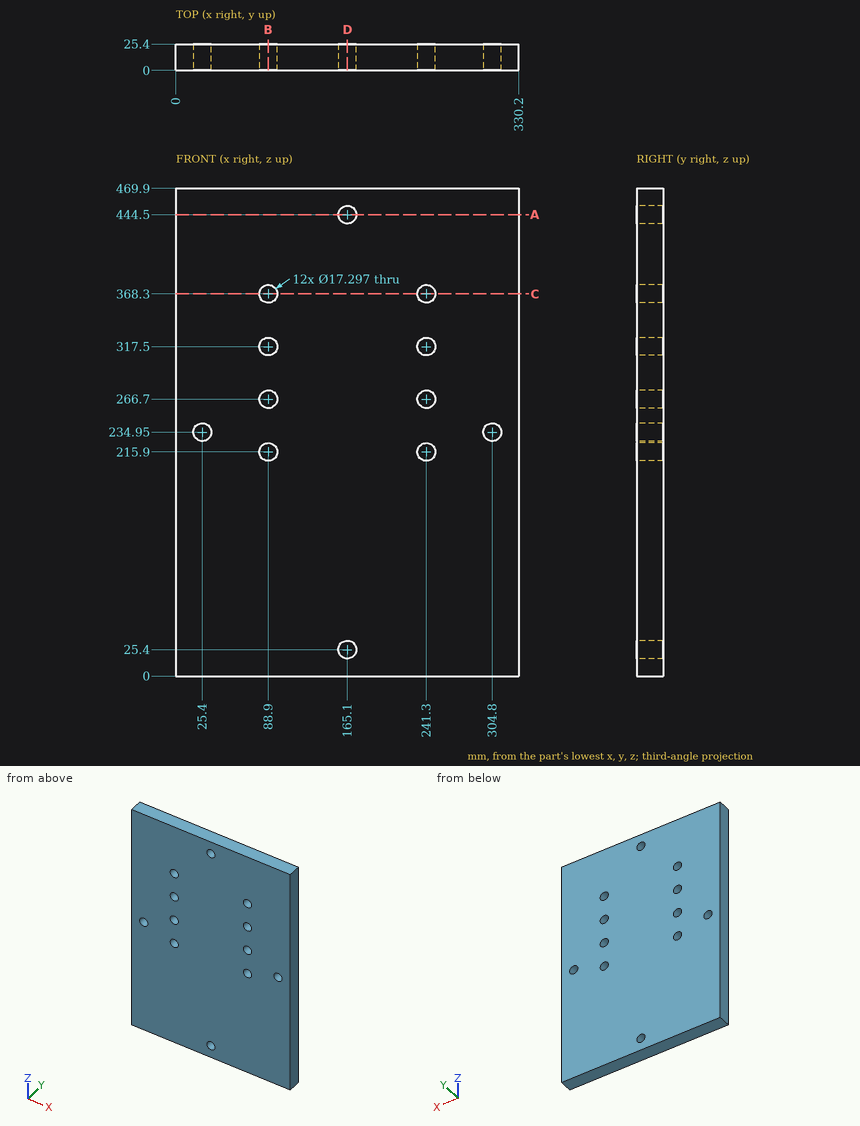
Geometry check sheet. Reference: drawing and pictorial views, mm from the part's lowest x, y, z. Round coordinates to 2 decimals unless told otherwise and drop trailing zeros. Order: outer loops, then holes, each group sorted by start corner. A loop starts at its lowest first (then second) coordinate and runs counter-clockwise, first axis right, second up. Notation, with made-up numbers: M 18.5,10.5 L 28.5,10.5 A27 cw 28.5,35.5 Z; hole C 74,-38 d4. An arc over 180 degrees is marked long. Answer in a Markdown table with one row per item.
(1) Go/stop test with flat-tipped pins: P1, Ø10.5, axis at x = 241.3, z = 215.9, coming from the +Y side; P2, Ø3, axis at x = 274.5, y = 20.5, coming from the -Z side. Record where each tip stops, or that it passes through.
Responses:
| item | result |
|---|---|
| P1 | passes through |
| P2 | stops at z = 0 |
(2) Sectioned sample at C-C, the plane z = 368.3. Record the cut outline in (x, y), and give its area (3 significant figures).
Responses:
| item | result |
|---|---|
| outline | M 0,0 L 80.25,0 L 80.25,25.4 L 0,25.4 Z; M 97.55,0 L 232.65,0 L 232.65,25.4 L 97.55,25.4 Z; M 249.95,0 L 330.2,0 L 330.2,25.4 L 249.95,25.4 Z |
| area | 7,510 mm² |
(3) Sectioned sample at A-A, the plane z = 444.5. Record the cut outline in (x, y), and give its area (3 significant figures).
Responses:
| item | result |
|---|---|
| outline | M 0,0 L 156.45,0 L 156.45,25.4 L 0,25.4 Z; M 173.75,0 L 330.2,0 L 330.2,25.4 L 173.75,25.4 Z |
| area | 7,950 mm² |
(4) Scan lines: probe 1 along X at (y, z) = (9.5, 368.3); probe 2 along X at (y, z) = (11.5, 234.95); probe 3 along X at (y, z) = (4.75, 444.5). Record each from-to range of solid material in increasing order. Write a range as from..to.
Responses:
| item | result |
|---|---|
| probe 1 | x = 0..80.25, 97.55..232.65, 249.95..330.2 |
| probe 2 | x = 0..16.75, 34.05..296.15, 313.45..330.2 |
| probe 3 | x = 0..156.45, 173.75..330.2 |
(5) Sectioned sample at B-B, the plane x = 88.9. Record the cut outline in (y, z).
Responses:
| item | result |
|---|---|
| outline | M 0,0 L 25.4,0 L 25.4,207.25 L 0,207.25 Z; M 0,224.55 L 25.4,224.55 L 25.4,258.05 L 0,258.05 Z; M 0,275.35 L 25.4,275.35 L 25.4,308.85 L 0,308.85 Z; M 0,326.15 L 25.4,326.15 L 25.4,359.65 L 0,359.65 Z; M 0,376.95 L 25.4,376.95 L 25.4,469.9 L 0,469.9 Z |
(6) Sectioned sample at D-D, the plane x = 165.1. Record the cut outline in (y, z).
Responses:
| item | result |
|---|---|
| outline | M 0,0 L 25.4,0 L 25.4,16.75 L 0,16.75 Z; M 0,34.05 L 25.4,34.05 L 25.4,435.85 L 0,435.85 Z; M 0,453.15 L 25.4,453.15 L 25.4,469.9 L 0,469.9 Z |
